Input: dimensioned drawing with shaded views. Units: mm. Origin: part minimum x, y, z. Give positions to 0.01 mm unless a question says otherwise; leave off trailing zeros. Write each loop counter-clockwise with the first axis right and the second up, starting at its lowest first coordinate (ties: lowest second). Pieces come first, ordered by that corner, then holes. Notation, with made-up numbers: (35, -2.5) -> (39, -2.5) arc R24 cw to (39, 9.5) -> close; hole circle Ø7 at (8, -22). An arc over 180 degrees is marked (long way). Return JSON: item names as keys, results as strings. Group by question number.
Item 1: Section C-C, the plane z = 144. Return loops of the section in (x, y), then the cut area to 3 significant figures.
Item 2: Pin query (flat end, axial travel): P1, Ø12, axis at x = 68, z = 404.5, coming from the +Y side; P2, Ø4, axis at y = 51, z = 336.5, coming from the -X side; P3, Ø6, axis at y = 65, z = 57, coming from the -X side. Return the tip coordinate at first contact, or that it passes through.
Item 3: Line query: line 1 (Y direction, x = 50, z = 197); line 2 (X direction, y = 51, z = 478.5); line 3 (Z direction, x = 69, y = 52). Output: solid intervals per line, ascending. Write a range as [from, to].
Item 4: Section B-B, the plane z = 86. Return loops of the section in (x, y).
Item 5: Section A-A, the plane x = 50. Return loops of the section in (y, z), then the cut area to 3 significant figures.
Item 6: Mould query, pull axis X, two halves, no side actions, for the marked faces 1, 2 and 3. Classes: released by +X, released by -X, zero draft, split by the parting line, or undercut.
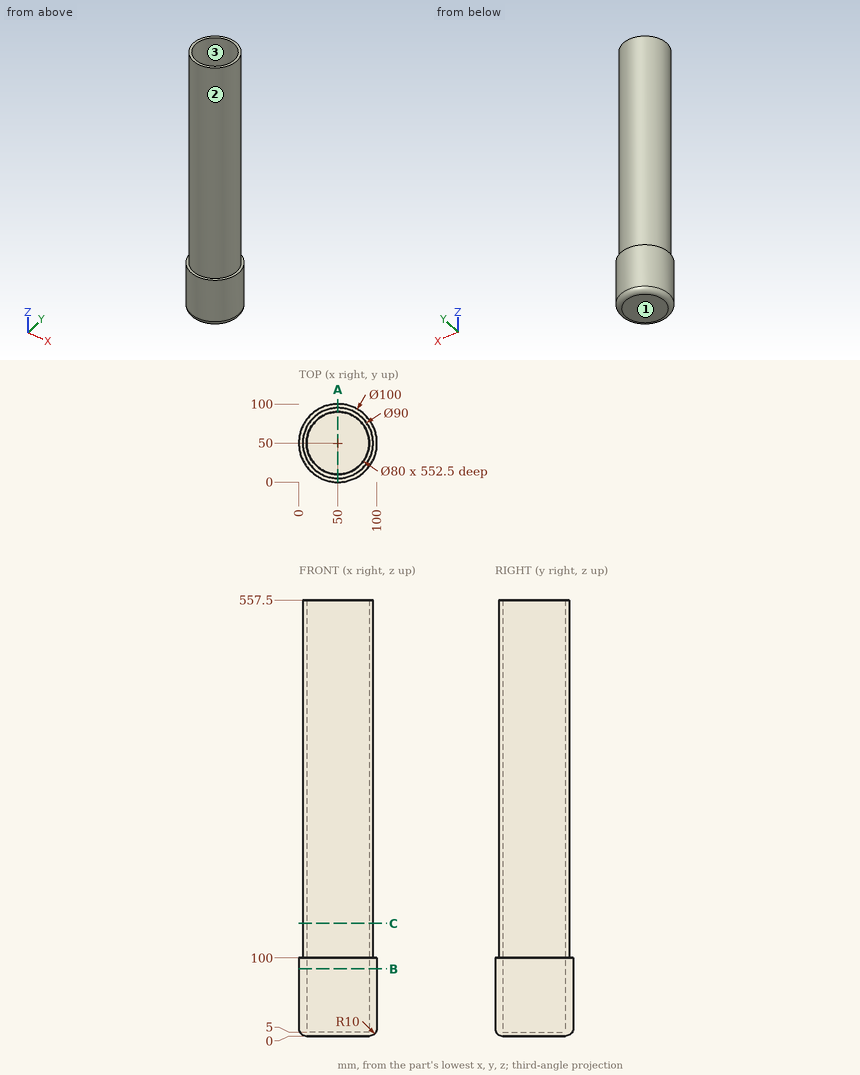
Answer below:
{
 "1": {"outline": "circle Ø90 at (50, 50); hole circle Ø80 at (50, 50)", "area": "1,340 mm2"},
 "2": {"P1": "stops at y = 93.37", "P2": "stops at x = 5", "P3": "stops at x = 1.46"},
 "3": {"line 1": "y = [5, 10], [90, 95]", "line 2": "x = [5.01, 10.01], [89.99, 94.99]", "line 3": "z = [0, 5]"},
 "4": {"outline": "circle Ø100 at (50, 50); hole circle Ø80 at (50, 50)"},
 "5": {"outline": "(0, 10) arc R10 ccw to (10, 0) -> (90, 0) arc R10 ccw to (100, 10) -> (100, 100) -> (95, 100) -> (95, 557.5) -> (90, 557.5) -> (90, 5) -> (10, 5) -> (10, 557.5) -> (5, 557.5) -> (5, 100) -> (0, 100) -> close", "area": "6,930 mm2"},
 "6": {"face 1": "zero draft", "face 2": "split by the parting line", "face 3": "undercut"}
}
